Geometry check sheet. Reference: drawing and pictorial views, mm from the part's lowest x, y, z. Give positions to 0.01 mm unless a question says otherwise; leave off trailing zeros. Loops run counter-clockwise (first coordinate to the right, second up) from the corner with the lowest first, then second, coordinate; pieces in that order, holes last. Notation, with made-up numbers: M 81.25,-22.5 L 105.25,-22.5 A17 cw 105.25,-10.5 Z; hole C 4.5,33 d11. An arc over 180 degrees is marked long. Use CSV: the item, a comma, the result in double quotes.
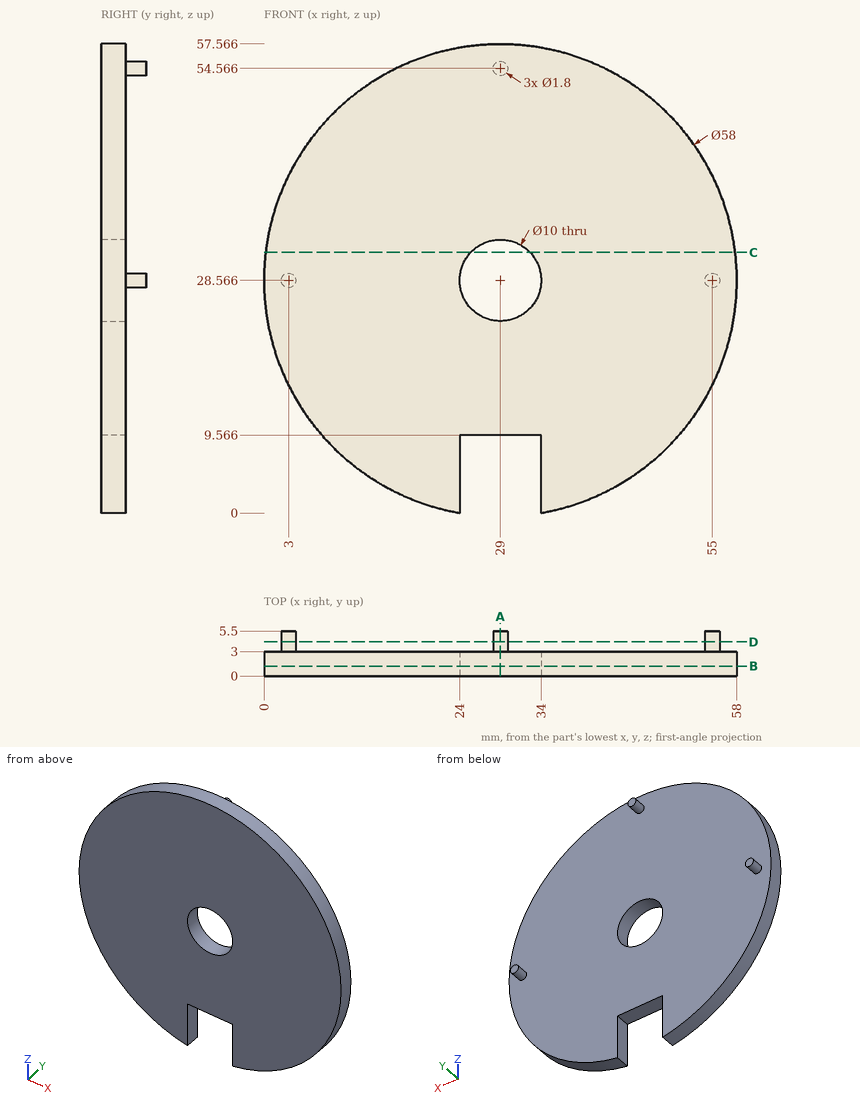
(1) Section check A-A on x = 29. Record the cut outline in (y, z).
Calculated:
outline,"M 0,9.57 L 3,9.57 L 3,23.57 L 0,23.57 Z; M 0,33.57 L 3,33.57 L 3,53.67 L 5.5,53.67 L 5.5,55.47 L 3,55.47 L 3,57.57 L 0,57.57 Z"
(2) Section check D-D on y = 4.2. Record the cut outline in (x, z).
Calculated:
outline,"C 3,28.57 d1.8; C 29,54.57 d1.8; C 55,28.57 d1.8"
(3) Scan lines: L1, parallel to Y at x = 38.5, z = 21; L2, parallel to X at y = 3.25, z = 29; L3, parallel to X at y = 2.5, z = 31. Record each from-to range of solid material in increasing order. Write a range as from..to.
Calculated:
L1,"y = 0..3"
L2,"x = 2.21..3.79, 54.21..55.79"
L3,"x = 0.1..24.63, 33.37..57.9"
(4) Section check B-B on y = 1.2. Record the cut outline in (x, z).
Calculated:
outline,"M 24,0 L 24,9.57 L 34,9.57 L 34,0 A29 ccw long Z; hole C 29,28.57 d10"
(5) Section check C-C on z = 32. Record the cut outline in (x, y).
Calculated:
outline,"M 0.2,0 L 25.37,0 L 25.37,3 L 0.2,3 Z; M 32.63,0 L 57.8,0 L 57.8,3 L 32.63,3 Z"
(6) Depth check by flat-ended pin: pin 1 Ø3 at (x, y) = (12.5, 2.5) entering from +Z (1 decimal); pin 2 Ø0.9 at (x, y) = (27.5, 2) entering from -Z; pin 3 Ø16 at (x, z) = (29, 28.57) entering from +Y; pin 4 Ø6 at (x, z) = (42, 37.5) entering from -Y. Enter the tip coordinate at first touch or a pass-through.
Calculated:
pin 1,"stops at z = 53.4"
pin 2,"stops at z = 9.57"
pin 3,"stops at y = 3"
pin 4,"stops at y = 0"
